Check sheet for the modelled part. Datum: model origin and axes. Units: mm. Coordinates: 2 decimals unless noted, no trailing zeros.
```python
from build123d import *

# Parameters (mm, degrees)
F0_W     = 68
F0_H     = 110
F0_R     = 1.5
F1_DEPTH = 4


with BuildPart() as f1:
    # F0 (on Top) → F1 (new body)
    with BuildSketch(Plane.XY):
        Rectangle(F0_W, F0_H)
        with Locations((-29, -50)):
            Circle(F0_R, mode=Mode.SUBTRACT)
        with Locations((-15, -15)):
            Circle(F0_R, mode=Mode.SUBTRACT)
        with BuildLine():
            ThreePointArc((30.5, -50), (27.9393398282, -51.0606601718), (29, -48.5))
            ThreePointArc((29, -48.5), (30.0606601718, -48.9393398282), (30.5, -50))
        make_face(mode=Mode.SUBTRACT)
        with BuildLine():
            ThreePointArc((16.5, -15), (13.9393398282, -16.0606601718), (15, -13.5))
            ThreePointArc((15, -13.5), (16.0606601718, -13.9393398282), (16.5, -15))
        make_face(mode=Mode.SUBTRACT)
        with Locations((-15, 15)):
            Circle(F0_R, mode=Mode.SUBTRACT)
        with Locations((-29, 50)):
            Circle(F0_R, mode=Mode.SUBTRACT)
        with BuildLine():
            ThreePointArc((15, 13.5), (13.9393398282, 13.9393398282), (13.5, 15))
            ThreePointArc((13.5, 15), (15, 16.5), (16.5, 15))
            ThreePointArc((16.5, 15), (16.0606601718, 13.9393398282), (15, 13.5))
        make_face(mode=Mode.SUBTRACT)
        with BuildLine():
            ThreePointArc((29, 48.5), (27.9393398282, 48.9393398282), (27.5, 50))
            ThreePointArc((27.5, 50), (29, 51.5), (30.5, 50))
            ThreePointArc((30.5, 50), (30.0606601718, 48.9393398282), (29, 48.5))
        make_face(mode=Mode.SUBTRACT)
    extrude(amount=F1_DEPTH)


solid = f1.part
```
1) Depth check by flat-ended pin: pin 1 (2.5 mm diameter, centred on x = 29, y = -50, fed in from +Z). Enter the tip coordinate at first touch or a pass-through.
Answer sheet:
pin 1: passes through
2) Scan lines: line 1 (Y direction, x = -29, z = 1.4); line 2 (Y direction, x = 15, z = 0.25); line 3 (X direction, y = 50.5, z = 3.5). Record each from-to range of solid material in increasing order.
Answer sheet:
line 1: y = -55 to -51.5, -48.5 to 48.5, 51.5 to 55
line 2: y = -55 to -16.5, -13.5 to 13.5, 16.5 to 55
line 3: x = -34 to -30.41, -27.59 to 27.59, 30.41 to 34
3) Mould release check, pull along X, two halves, no side actions. Record for faces 1 (the flat face through (0, -55, 2)), 2 (the flat face through (-34, -1, 2)), 3 (the cylindrical face through (-16.5, -14.93, 1.97)): +X half, -X half, draft (parallel to the pull), parting line (faces both ways), or undercut.
Answer sheet:
face 1: draft
face 2: -X half
face 3: undercut
